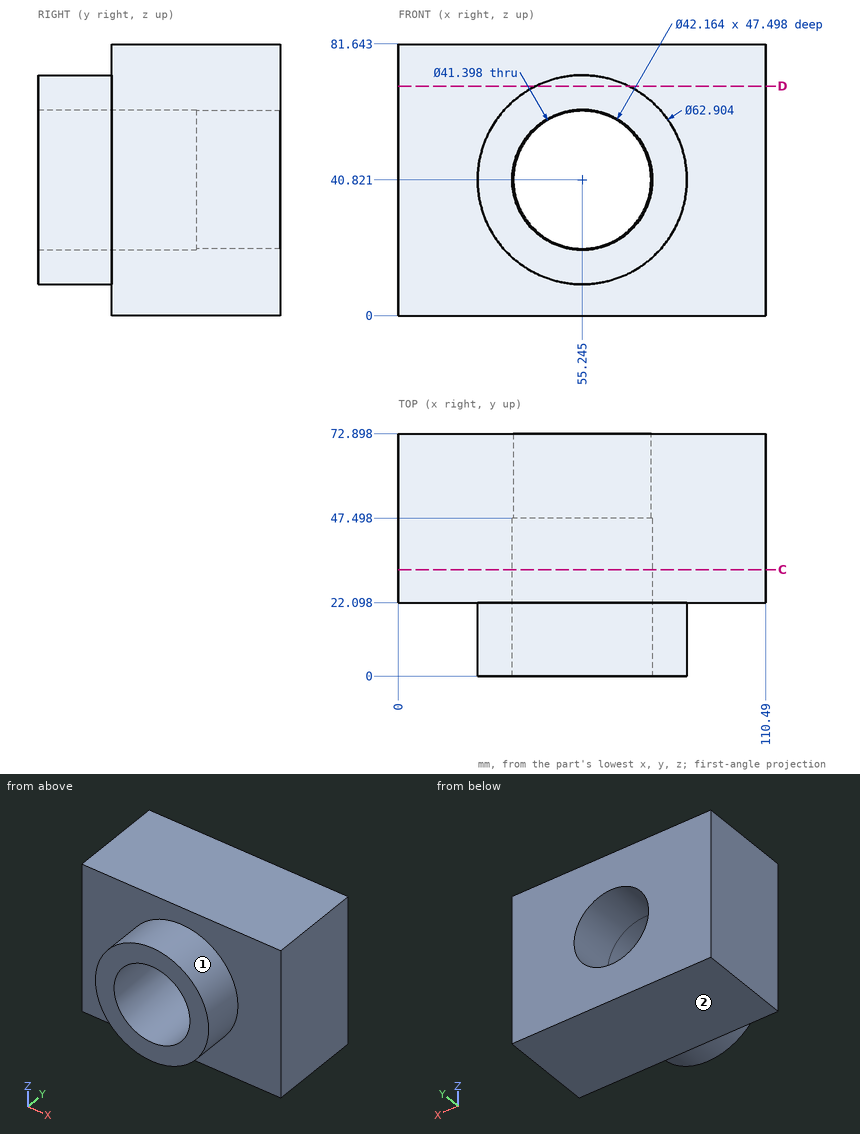
Print and shaded views of the part. All mm, measured from the part's lowest x, y and z. A direction names the side the tool comes from. Give positions to 0.01 mm unless a question says otherwise; leave off trailing zeros. Write each loop counter-clockwise with the first axis right and the second up, starting at its lowest first coordinate (ties: lowest second). Pieces come first, ordered by that corner, then holes. Notation, with made-up numbers: (-38.5, -25.75) - (12.5, -25.75) arc R24 cw to (12.5, 6.25) - close; hole circle Ø7 at (25.25, 10.25). An arc over 180 degrees is marked (long way). One line per question, with ' | ' between items. Start each with the question number.
(1) Slice it at D-D on z = 69. Write the cut outline in (x, y).
(2) Slice it at C-C on y = 32. Write the cut outline in (x, z) (1 decimal), plus the area to 3 significant figures.
(3) Pin check, flat tips, straight feed: P1, Ø3, axis at y = 12, z = 61, coming from the +X side; P2, Ø3, axis at y = 16.5, z = 71.5, coming from the +X side (1 decimal); P3, Ø25, axis at x = 55.25, z = 40.82, coming from the -Y side; P4, Ø1, axis at y = 20, z = 40.5, coming from the +X side. Stop position of each tip, or through.
(4) 3-axis set-ups, long thin cutter, end or side, ignore diameter. For the marked faces 1 and 2: which of +Z, -Z, +X, -X, +Y, -Y reach the whole face in a straight line?
(5) Wall check: line 1 along Y through (x, z) = (96.5, 65); line 2 along X through (y, z) = (22, 36.5); line 3 along Z through (x, y) = (51.5, 62.5) (1 decimal). Give the ranges that are in metal, low to high. Write a range as from..to.
Results below:
1) outline: (0, 22.1) - (41.27, 22.1) - (41.27, 0) - (69.22, 0) - (69.22, 22.1) - (110.49, 22.1) - (110.49, 72.9) - (0, 72.9) - close
2) outline: (0, 0) - (110.5, 0) - (110.5, 81.6) - (0, 81.6) - close; hole circle Ø42.2 at (55.2, 40.8) | area: 7,620 mm^2
3) P1: x = 80.55 | P2: x = 67 | P3: through | P4: x = 86.7
4) face 1: -Y | face 2: -Z, +X, -X, +Y, -Y
5) line 1: 22.1..72.9 | line 2: 24.09..34.61, 75.88..86.4 | line 3: 0..20.5, 61.2..81.6
